```python
from build123d import *

# Parameters (mm, degrees)
BOSS_EXTRUDE1_DEPTH = 15
SKETCH2_W           = 10.1
SKETCH2_H           = 10.1
CUT_EXTRUDE1_DEPTH  = 20
SKETCH3_W           = 10.1
SKETCH3_H           = 10.1
CUT_EXTRUDE2_DEPTH  = 17
SKETCH4_W           = 8
SKETCH4_H           = 8
CUT_EXTRUDE3_DEPTH  = 4
CUT_EXTRUDE4_REACH  = 41.051
SKETCH5_W           = 8
SKETCH5_H           = 8
FILLET1_R           = 5


with BuildPart() as part:
    # Sketch1 → Boss-Extrude1 (new body)
    with BuildSketch(Plane(origin=(0, 0, 0), x_dir=(1, 0, 0), z_dir=(0, 1, 0))):
        Polygon((0, 0), (20, 0), (20, 15), (0, 15), (0, 30), (-15, 30), (-15, 0), align=None)
    extrude(amount=BOSS_EXTRUDE1_DEPTH)

    # Sketch2 → Cut-Extrude1 (cut)
    with BuildSketch(Plane(origin=(20, 0, 0), x_dir=(0, 0, -1), z_dir=(1, 0, 0))):
        with Locations((7.5, 7.5)):
            Rectangle(SKETCH2_W, SKETCH2_H)
    extrude(amount=-CUT_EXTRUDE1_DEPTH, mode=Mode.SUBTRACT)

    # Sketch3 → Cut-Extrude2 (cut)
    with BuildSketch(Plane(origin=(0, 0, -30), x_dir=(-1, 0, 0), z_dir=(0, 0, -1))):
        with Locations((7.5, 7.5)):
            Rectangle(SKETCH3_W, SKETCH3_H)
    extrude(amount=-CUT_EXTRUDE2_DEPTH, mode=Mode.SUBTRACT)

    # Sketch4 → Cut-Extrude3 (cut)
    with BuildSketch(Plane(origin=(0, 0, -13), x_dir=(-1, 0, 0), z_dir=(0, 0, -1))):
        with Locations((7.5, 7.5)):
            Rectangle(SKETCH4_W, SKETCH4_H)
    extrude(amount=-CUT_EXTRUDE3_DEPTH, mode=Mode.SUBTRACT)

    # Cut-Extrude4: up to this face of the body (flat: up to its plane)
    cut_extrude4_end = Plane(part.part.faces().sort_by_distance((-11.5, 7.5, -11))[0])
    # Sketch5 → Cut-Extrude4 (cut, up to the picked face)
    with BuildSketch(Plane(origin=(0, 0, 0), x_dir=(0, 0, -1), z_dir=(1, 0, 0)), mode=Mode.PRIVATE) as cut_extrude4_sk1:
        with Locations((7.5, 7.5)):
            Rectangle(SKETCH5_W, SKETCH5_H)
    cut_extrude4_tool1 = split(extrude(cut_extrude4_sk1.sketch, amount=-CUT_EXTRUDE4_REACH, mode=Mode.PRIVATE), bisect_by=cut_extrude4_end, keep=Keep.BOTH, mode=Mode.PRIVATE)
    add(cut_extrude4_tool1.solids().sort_by(Axis((0, 7.5, -7.5), (-1, 0, 0)))[0], mode=Mode.SUBTRACT)

    # Fillet1
    # the kernel refuses this fillet: 5 mm, written as the material it adds along each edge
    with BuildSketch(Plane(origin=(-11.5, -9, -3.5), x_dir=(1, 0, 0), z_dir=(0, 1, 0))) as fillet1_piece_1_section:
        with BuildLine():
            CenterArc((FILLET1_R, FILLET1_R), FILLET1_R, 180, 90)
            Line((0, FILLET1_R), (0, 0))
            Line((0, 0), (FILLET1_R, 0))
        make_face()
    fillet1_piece_1 = extrude(amount=20.5, mode=Mode.PRIVATE)
    fillet1_piece_1 = split(fillet1_piece_1, bisect_by=Plane(origin=(-11.5, 0, -3.5), z_dir=(0, 1, 0)), keep=Keep.TOP, mode=Mode.PRIVATE)
    add(fillet1_piece_1)
    # the kernel refuses this fillet: 5 mm, written as the material it takes off along each edge
    with BuildSketch(Plane(origin=(-3.5, 3.5, -11.5), x_dir=(1, 0, 0), z_dir=(0, 1, 0))) as fillet1_2_piece_1:
        with BuildLine():
            CenterArc((3.570714214, 5), FILLET1_R, 224.427004001, 45.572995999)
            Line((0, 1.5), (0, 0))
            Line((0, 0), (3.570714214, 0))
        make_face()
    extrude(amount=8, mode=Mode.SUBTRACT)


solid = part.part
```
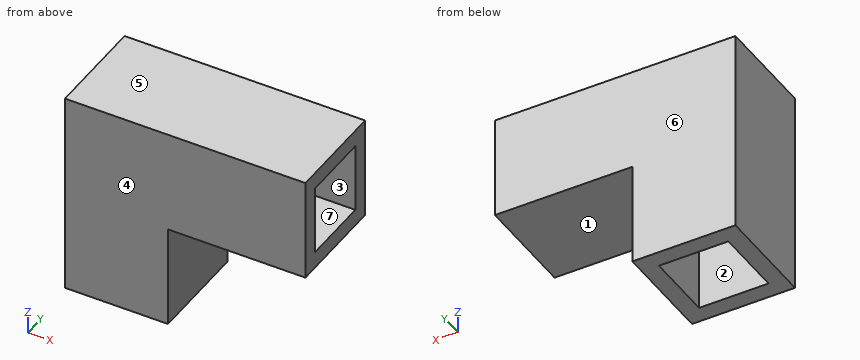
Geometry check sheet. Reference: the model listing, model coordinates, mm. Face numbers are marked on the shaded views. A direction names the side the tool comes from. Round coordinates to 2 decimals unless told otherwise and drop trailing zeros. Loops run counter-clockwise (first coordinate to the right, second up) from the corner with the lowest first, then second, coordinate; pieces in that order, holes last. Notation, with made-up numbers: (19.5, 45.5) - (71.5, 45.5) arc R14 cw to (71.5, 62.5) - close; hole circle Ø6 at (85, 74). An arc over 180 degrees is marked (long way). Write each question's results on one line, items separated by ' | '. Start each with the question number.
Q1. Cross-section at D-D on z = -3. Enter the section's corners in (x, y), and give its area (3 significant figures).
Q2. Cross-section at C-C on x = 8.5. Enter the section's corners in (y, z), and give its area (3 significant figures).
Q3. Gauge pin test, flat ends, axial feed: P1, Ø3, axis at y = 12.5, z = -19, coming from the +X side; P2, Ø4, axis at x = 15.5, y = 3, coming from the -Z side. Record the tip position at first contact, or that the pin passes through.
Q4. Thickness scan on line 1 (Z direction, x = 5, y = 5.75); line 2 (Y direction, x = 11, z = -6.5). Record the ranges inside material, lowest first. Write a range as [from, to].
Q5. Release check for a two-part mould opening along Y. For the marked faces 5, 6 and 7 record: +Y half, -Y half, draft (parallel to the pull), parting line (faces both ways), or undercut.
Q6. Cross-section at B-B on z = -18. Enter the section's corners in (x, y), and give its area (3 significant figures).
Q7. Access from +Z, -Z, +X, -X, +Y, -Y to the whole of each face (thin tool, end or side, straight path). Record for the marked faces 1, 2, 3 and 4.
Q8. Cross-section at A-A on y = 5. Enter the section's corners in (x, z).
Answers below:
1) outline: (-15, 0) - (20, 0) - (20, 2.45) - (0, 2.45) - (0, 12.55) - (20, 12.55) - (20, 15) - (-15, 15) - close | area: 323 mm²
2) outline: (0, -15) - (15, -15) - (15, 0) - (0, 0) - close; hole (2.45, -12.55) - (12.55, -12.55) - (12.55, -2.45) - (2.45, -2.45) - close | area: 123 mm²
3) P1: stops at x = 0 | P2: stops at z = -15
4) line 1: z = [-15, -12.55], [-2.45, 0] | line 2: y = [0, 2.45], [12.55, 15]
5) face 5: draft | face 6: +Y half | face 7: undercut
6) outline: (-15, 0) - (0, 0) - (0, 15) - (-15, 15) - close; hole (-12.55, 2.45) - (-2.45, 2.45) - (-2.45, 12.55) - (-12.55, 12.55) - close | area: 123 mm²
7) face 1: -Z, +X, +Y, -Y | face 2: -Z | face 3: +X | face 4: +Z, -Z, +X, -X, -Y
8) outline: (-15, -30) - (-12.55, -30) - (-12.55, -13) - (-11.5, -13) - (-11.5, -8.5) arc R5 cw to (-6.5, -3.5) - (0, -3.5) - (0, -2.45) - (20, -2.45) - (20, 0) - (-15, 0) - close; (-3.5, -13) - (-2.45, -13) - (-2.45, -30) - (0, -30) - (0, -15) - (20, -15) - (20, -12.55) - (0, -12.55) - (0, -11.5) arc R5 ccw to start
